Can you work these out from the model? Positions are in its coordinate system, mm. Give positions to 0.01 mm unless a question says otherwise; leave off trailing zeros. Order: outer loops, then holes, each group sorted by start corner. A loop starts at its lowest first (then second) coordinate and runs counter-clockwise, first axis right, second up.
Item 1: I want a section at B-B, the plane y = 106.5. Write out the boundary of the cut face in (x, z), then the cut area to 3 significant figures.
Item 2: I want a section at C-C, the plane z = 8.75. Write out the boundary of the cut face in (x, y), then the cut area to 3 significant figures.
Item 3: If I drill on line 1 along X through (y, z) = (-56.5, 5.5); line 2 along X through (y, z) = (-124.5, 6.75); line 3 along Y through (x, z) = (-1.5, 12), over which ranges is the centre line in solid material (lowest first)?
Item 4: I want a section at D-D, the plane x = -111. Write out the boundary of the cut face in (y, z), then the cut area to 3 significant figures.
Item 5: I'm going to push flat-ended pins straight in: pin 1 Ø3 at (y, z) = (-5.5, 7) entering from -X; pin 2 Ø6.5 at (y, z) = (176.5, 6) entering from +X; pin 3 Ø3 at (x, z) = (-97.5, 6.5) entering from -Y. Where does each tip first touch, or does it pass through?
Item 6: I want a section at A-A, the plane x = 110.5. Write out the boundary of the cut face in (y, z), then the cut area to 3 significant figures.
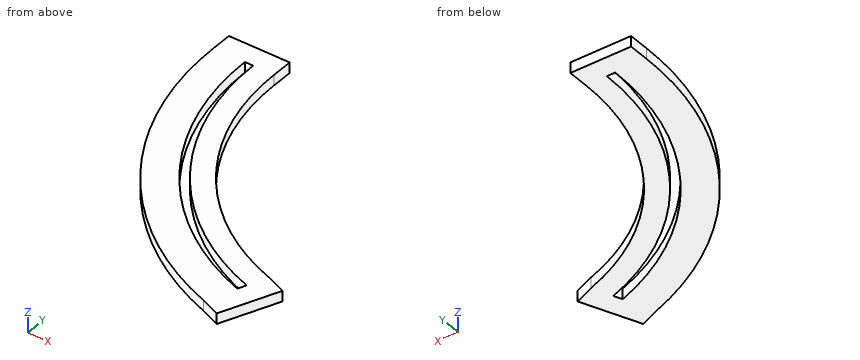
```python
from build123d import *

# Parameters (mm, degrees)
F1_DEPTH = 12.7


with BuildPart() as f1:
    # F0 (on Top) → F1 (new body)
    with BuildSketch(Plane.XY):
        with BuildLine():
            ThreePointArc((129.422316, -115.545373), (-12.974184, -10.525769), (-67.249111, 157.878841))
            Line((-67.249111, 157.878841), (-67.249111, 183.278841))
            Line((-67.249111, 183.278841), (-140.909111, 183.278841))
            Line((-140.909111, 183.278841), (-140.909111, 157.878841))
            ThreePointArc((-140.909111, 157.878841), (-74.536341, -51.212117), (100.278697, -183.741644))
            Line((100.278697, -183.741644), (123.635304, -193.723071))
            Line((123.635304, -193.723071), (152.778923, -125.5268))
            Line((152.778923, -125.5268), (129.422316, -115.545373))
        make_face()
        with BuildLine():
            Line((-102.809111, 157.878841), (-92.649111, 157.878841))
            ThreePointArc((-92.649111, 157.878841), (-34.176979, -24.508812), (119.440889, -138.901981))
            Line((119.440889, -138.901981), (115.250837, -148.706732))
            ThreePointArc((115.250837, -148.706732), (-42.734212, -30.233396), (-102.809111, 157.878841))
        make_face(mode=Mode.SUBTRACT)
    extrude(amount=F1_DEPTH)


solid = f1.part
```
Results list:
1. outline: (-137.25, 0) - (-98.72, 0) - (-98.72, 12.7) - (-137.25, 12.7) - close; (-88.41, 0) - (-62.64, 0) - (-62.64, 12.7) - (-88.41, 12.7) - close
1. area: 817 mm2
2. outline: (-140.91, 157.88) arc R362.53 ccw to (100.28, -183.74) - (123.64, -193.72) - (152.78, -125.53) - (129.42, -115.55) arc R288.4 cw to (-67.25, 157.88) - (-67.25, 183.28) - (-140.91, 183.28) - close; hole (-102.81, 157.88) arc R324.55 ccw to (115.25, -148.71) - (119.44, -138.9) arc R313.69 cw to (-92.65, 157.88) - close
2. area: 29,400 mm2
3. line 1: x = -70.73 to -21.93, -7.96 to 28.24
3. line 2: x = -5.73 to 61.75, 84.43 to 150.38
3. line 3: y = -127.86 to -77.7, -63.2 to -25.43
4. outline: (13.69, 0) - (183.28, 0) - (183.28, 12.7) - (13.69, 12.7) - close
4. area: 2,150 mm2
5. pin 1: stops at x = -102.76
5. pin 2: stops at x = -67.25
5. pin 3: stops at y = -16.89
6. outline: (-188.11, 0) - (-147.02, 0) - (-147.02, 12.7) - (-188.11, 12.7) - close; (-135.69, 0) - (-108.45, 0) - (-108.45, 12.7) - (-135.69, 12.7) - close
6. area: 868 mm2
